from build123d import *

# Parameters (mm, degrees)
SKETCH_1_W          = 94
SKETCH_1_H          = 100
SKETCH_1_R          = 3
SKETCH_1_W_2        = 50
SKETCH_1_H_2        = 12
EXTRUDE_1_DEPTH     = 12
SKETCH_2_R          = 5.5
CUT_EXTRUDE_1_DEPTH = 6
SKETCH_3_R          = 3
CUT_EXTRUDE_2_DEPTH = 10


with BuildPart() as part:
    # 草图1 → 凸台-拉伸1 (new body)
    with BuildSketch(Plane.XY):
        Rectangle(SKETCH_1_W, SKETCH_1_H)
        with Locations((10, 44)):
            Circle(SKETCH_1_R, mode=Mode.SUBTRACT)
        with Locations((-10, 44)):
            Circle(SKETCH_1_R, mode=Mode.SUBTRACT)
        with Locations((-41, -35)):
            Circle(SKETCH_1_R, mode=Mode.SUBTRACT)
        with Locations((-41, -15)):
            Circle(SKETCH_1_R, mode=Mode.SUBTRACT)
        with Locations((-41, 5)):
            Circle(SKETCH_1_R, mode=Mode.SUBTRACT)
        with Locations((-41, 25)):
            Circle(SKETCH_1_R, mode=Mode.SUBTRACT)
        with Locations(Location((41, -35, 0), (0, 0, 180))):
            Circle(SKETCH_1_R, mode=Mode.SUBTRACT)
        with Locations(Location((41, -15, 0), (0, 0, 180))):
            Circle(SKETCH_1_R, mode=Mode.SUBTRACT)
        with Locations(Location((41, 5, 0), (0, 0, 180))):
            Circle(SKETCH_1_R, mode=Mode.SUBTRACT)
        with Locations(Location((41, 25, 0), (0, 0, 180))):
            Circle(SKETCH_1_R, mode=Mode.SUBTRACT)
        with Locations((-9, 14.5)):
            Circle(SKETCH_1_R, mode=Mode.SUBTRACT)
        with Locations((9, 14.5)):
            Circle(SKETCH_1_R, mode=Mode.SUBTRACT)
        with Locations((0, 26.5)):
            Rectangle(SKETCH_1_W_2, SKETCH_1_H_2, mode=Mode.SUBTRACT)
    extrude(amount=EXTRUDE_1_DEPTH)

    # 草图2 → 切除-拉伸1 (cut)
    with BuildSketch(Plane.XY.offset(12)):
        with Locations((-10, 44)):
            Circle(SKETCH_2_R)
        with Locations((-41, 25)):
            Circle(SKETCH_2_R)
        with Locations((-41, 5)):
            Circle(SKETCH_2_R)
        with Locations((-41, -15)):
            Circle(SKETCH_2_R)
        with Locations(Location((41, -35, 0), (0, 0, 180))):
            Circle(SKETCH_2_R)
        with Locations((-41, -35)):
            Circle(SKETCH_2_R)
        with Locations(Location((41, -15, 0), (0, 0, 180))):
            Circle(SKETCH_2_R)
        with Locations(Location((41, 5, 0), (0, 0, 180))):
            Circle(SKETCH_2_R)
        with Locations(Location((41, 25, 0), (0, 0, 180))):
            Circle(SKETCH_2_R)
        with Locations(Location((10, 44, 0), (0, 0, 180))):
            Circle(SKETCH_2_R)
    extrude(amount=-CUT_EXTRUDE_1_DEPTH, mode=Mode.SUBTRACT)

    # 草图3 → 切除-拉伸2 (cut)
    with BuildSketch(Plane.XZ.offset(50)):
        with Locations(Location((-33, 6, 0), (0, 0, 270))):
            Circle(SKETCH_3_R)
        with Locations(Location((-8, 6, 0), (0, 0, 270))):
            Circle(SKETCH_3_R)
        with Locations(Location((33, 6, 0), (0, 0, 90))):
            Circle(SKETCH_3_R)
        with Locations(Location((8, 6, 0), (0, 0, 90))):
            Circle(SKETCH_3_R)
    extrude(amount=-CUT_EXTRUDE_2_DEPTH, mode=Mode.SUBTRACT)


solid = part.part
The listing builds one solid part. Answer for the finished solid, in the listing's coordinates (mm). A direction names the side the tool comes from. Coordinates: 2 decimals unless noted, no trailing zeros. Order: outer loops, then holes, each group sorted by start corner. A loop starts at its lowest first (then second) coordinate and runs counter-clockwise, first axis right, second up.
Q1. Given P1, Ø5.5, axis at x = -42, y = 5, coming from the +Z side; P2, Ø1.8, axis at x = 34, z = 7, coming from the -Y side, each flat-ended and moving along its own axis, determine where each tip first touches the part or whether it passes through.
Q2. A cutting plane is placed at C-C, the plane z = 1.5. State how many separate pieces and enclosed holes the cut face has, and give its area (3 significant figures).
Q3. A cutting plane is placed at B-B, the plane x = 17. Write down the section's boundary in (y, z).
Q4. Consider line 1 (X direction, y = 25, z = 2.55); line 2 (Y direction, x = -41, z = 9); line 3 (Z direction, x = 8, y = -42). Determine where each line is inside the solid, lowest interval first.
Q5. Which of the six approach directions +Z, -Z, +X, -X, +Y, -Y give full straight-line access (tool end or side, diameter ignored) to faces 1 (the face through (-1, -50, 6)), 2 (the face through (25, 26, 6)), 3 (the face through (5.47, -45.07, 7.61)), 4 (the face through (-46.495, 5.242, 9.042))?
Q6. For a pull along Z with two mould halves and no side action, classify faces 5 (the face through (44, 5, 3)), 6 (the face through (38.6, 27.4, 6)), 7 (the face through (35.662, -45.07, 7.384)), 8 (the face through (-33, -40, 6)) as pulls with the +Z half, pulls with the -Z half, needs draft (parallel to the pull), parting line crosses it, or undercut.
Q7. A cutting plane is placed at D-D, the plane x = -33. Write down the section's boundary in (y, z).
Q8. A cutting plane is placed at A-A, the plane y = -35. Write down the section's boundary in (x, z), and give its area (3 significant figures).
Answers follow:
1. P1: stops at z = 6
1. P2: stops at y = -40
2. separate pieces: 1
2. enclosed holes: 13
2. area: 8,460 mm2
3. outline: (-50, 0) - (20.5, 0) - (20.5, 12) - (-50, 12) - close; (32.5, 0) - (50, 0) - (50, 12) - (32.5, 12) - close
4. line 1: x = -47 to -44, -38 to -25, 25 to 38, 44 to 47
4. line 2: y = -50 to -40.5, -29.5 to -20.5, -9.5 to -0.5, 10.5 to 19.5, 30.5 to 50
4. line 3: z = 0 to 3, 9 to 12
5. face 1: +Z, -Z, +X, -X, -Y
5. face 2: +Z, -Z
5. face 3: -Y
5. face 4: +Z
6. face 5: needs draft
6. face 6: pulls with the +Z half
6. face 7: undercut
6. face 8: undercut
7. outline: (-50, 0) - (50, 0) - (50, 12) - (-50, 12) - (-50, 9) - (-40, 9) - (-40, 3) - (-50, 3) - close
8. outline: (-47, 0) - (-44, 0) - (-44, 6) - (-46.5, 6) - (-46.5, 12) - (-47, 12) - close; (-38, 0) - (38, 0) - (38, 6) - (35.5, 6) - (35.5, 12) - (-35.5, 12) - (-35.5, 6) - (-38, 6) - close; (44, 0) - (47, 0) - (47, 12) - (46.5, 12) - (46.5, 6) - (44, 6) - close
8. area: 924 mm2
